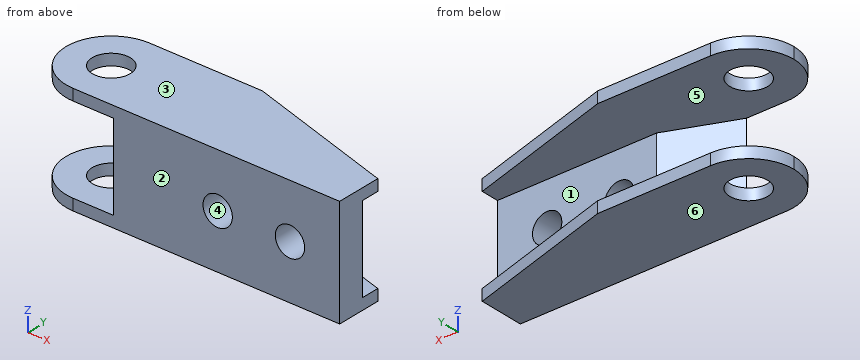
```python
from build123d import *

# Parameters (mm, degrees)
CROQUIS1_W              = 34.5
CROQUIS1_H              = 12
SALIENTE_EXTRUIR1_DEPTH = 10
REDONDEO1_R             = 5
CROQUIS8_W              = 34.5
CROQUIS8_H              = 9.5
CORTAR_EXTRUIR6_DEPTH   = 7
CROQUIS9_W              = 10.737065785
CROQUIS9_H              = 9.5
CORTAR_EXTRUIR7_DEPTH   = 21.822163672
CHAFL_N1_SIZE           = 3
CHAFL_N1_SIZE_2         = 7.42526056
CORTAR_EXTRUIR8_DEPTH   = 24.27149544
CROQUIS11_R             = 2.1
CORTAR_EXTRUIR9_DEPTH   = 24.27149544
CROQUIS12_R             = 1.625
CORTAR_EXTRUIR10_DEPTH  = 20.559204994


# Some blends are built 0.0001 mm under size
with BuildPart() as part:
    # Croquis1 → Saliente-Extruir1 (new body)
    with BuildSketch(Plane(origin=(0, 0, 0), x_dir=(1, 0, 0), z_dir=(0, 1, 0))):
        Rectangle(CROQUIS1_W, CROQUIS1_H)
    extrude(amount=SALIENTE_EXTRUIR1_DEPTH)

    # Redondeo1
    redondeo1_edges = [part.edges().sort_by_distance(p)[0] for p in [
        (-17.25, 10, 0),
        (-17.25, 0, 0),
    ]]
    fillet(redondeo1_edges, radius=REDONDEO1_R - 0.0001)  # a hair under: the kernel refuses the full size

    # Croquis8 → Cortar-Extruir6 (cut)
    with BuildSketch(Plane(origin=(0, 10, 0), x_dir=(1, 0, 0), z_dir=(0, 1, 0))):
        Rectangle(CROQUIS8_W, CROQUIS8_H)
    extrude(amount=-CORTAR_EXTRUIR6_DEPTH, mode=Mode.SUBTRACT)

    # Croquis9 → Cortar-Extruir7 (cut, through all)
    with BuildSketch(Plane.XZ):
        with Locations((-13.168532893, 0)):
            Rectangle(CROQUIS9_W, CROQUIS9_H)
    extrude(amount=-CORTAR_EXTRUIR7_DEPTH, mode=Mode.SUBTRACT)

    # Chaflán1
    # the kernel refuses this chamfer: 7.42526056, 3 mm, written as the material it takes off along each edge
    with BuildSketch(Plane(origin=(-7.8, 3, -4.75), x_dir=(-0.08816706473193606, -0.9961057015681392, 0), z_dir=(0, 0, 1))) as chafl_n1_piece_1:
        Polygon((CHAFL_N1_SIZE * 0.996105701568, CHAFL_N1_SIZE * 0.0881670647319), (-CHAFL_N1_SIZE_2 * 0.0881670647349, CHAFL_N1_SIZE_2 * 0.996105701602), (0, 0), align=None)
    extrude(amount=9.5, mode=Mode.SUBTRACT)

    # Croquis10 → Cortar-Extruir8 (cut, through all)
    with BuildSketch(Plane.XY.offset(6)):
        Polygon((0.25, 10), (17.25, 5), (17.25, 10), align=None)
    extrude(amount=-CORTAR_EXTRUIR8_DEPTH, mode=Mode.SUBTRACT)

    # Croquis11 → Cortar-Extruir9 (cut, through all)
    with BuildSketch(Plane.XY.offset(6)):
        with Locations((-12.25, 5)):
            Circle(CROQUIS11_R)
    extrude(amount=-CORTAR_EXTRUIR9_DEPTH, mode=Mode.SUBTRACT)

    # Croquis12 → Cortar-Extruir10 (cut, through all)
    with BuildSketch(Plane(origin=(0, 3, 0), x_dir=(1, 0, 0), z_dir=(0, 1, 0))):
        with Locations(Location((3.75, 0, 0), (0, 0, 270))):
            Circle(CROQUIS12_R)
        with Locations(Location((11.75, 0, 0), (0, 0, 270))):
            Circle(CROQUIS12_R)
    extrude(amount=-CORTAR_EXTRUIR10_DEPTH, mode=Mode.SUBTRACT)


solid = part.part
```
Geometry check sheet. Reference: the model listing, model coordinates, mm. Face numbers are marked on the shaded views. A direction names the side the tool comes from. Give positions to 0.01 mm unless a question says otherwise; leave off trailing zeros. Write each loop counter-clockwise with the first axis right and the second up, starting at its lowest first coordinate (ties: lowest second). Pieces come first, ordered by that corner, then holes. Notation, with made-up numbers: (-32.5, 11) - (23.5, 11) arc R23 ccw to (23.5, 43) - close; hole circle Ø7 at (32.5, 35). An arc over 180 degrees is marked (long way). Use a Markdown table: item, result.
Q1. Draft check along Z on the marked faces 1, 2, 3 and 4. Enter one of: pulls with the +Z half, pulls with the -Z half, needs draft (parallel to the pull), parting line crosses it, or undercut.
Computed:
| item | result |
|---|---|
| face 1 | undercut |
| face 2 | needs draft |
| face 3 | pulls with the +Z half |
| face 4 | undercut |
Q2. Section check A-A, the plane z = 0. Enter the section's corners in (x, y) (3 decimals), then the cut area to 3 significant figures.
Computed:
| item | result |
|---|---|
| outline | (-7.8, 0) - (2.125, 0) - (2.125, 3) - (-0.375, 3) - close; (5.375, 0) - (10.125, 0) - (10.125, 3) - (5.375, 3) - close; (13.375, 0) - (17.25, 0) - (17.25, 3) - (13.375, 3) - close |
| area | 44.5 mm² |
Q3. Go/stop test with flat-tipped pins: P1, Ø6, axis at x = 6.5, z = 2, coming from the -Y side; P2, Ø3, axis at y = 8, z = -4.5, coming from the -X side; P3, Ø3, axis at x = 6, z = 2, coming from the +Y side. Record where each tip stops, or that it passes through.
Computed:
| item | result |
|---|---|
| P1 | stops at y = 0 |
| P2 | stops at x = -17.01 |
| P3 | stops at y = 3 |
Q4. Section check C-C, the plane y = 8.5. Enter the section's corners in (x, z).
Computed:
| item | result |
|---|---|
| outline | (-15.82, -6) - (5.35, -6) - (5.35, -4.75) - (-15.82, -4.75) - close; (-15.82, 4.75) - (5.35, 4.75) - (5.35, 6) - (-15.82, 6) - close |
Q5. Section check D-D, the plane y = 4.25. Enter the section's corners in (x, z).
Computed:
| item | result |
|---|---|
| outline | (-17.19, -6) - (-14.21, -6) - (-14.21, -4.75) - (-17.19, -4.75) - close; (-17.19, 4.75) - (-14.21, 4.75) - (-14.21, 6) - (-17.19, 6) - close; (-10.29, -6) - (17.25, -6) - (17.25, -4.75) - (-10.29, -4.75) - close; (-10.29, 4.75) - (17.25, 4.75) - (17.25, 6) - (-10.29, 6) - close |
Q6. Section check B-B, the plane x = -8.5. Enter the section's corners in (y, z), then the cut area to 3 significant figures.
Computed:
| item | result |
|---|---|
| outline | (0, -6) - (10, -6) - (10, -4.75) - (0, -4.75) - close; (0, 4.75) - (10, 4.75) - (10, 6) - (0, 6) - close |
| area | 25.0 mm² |
Q7. Thickness scan on L1, parallel to Y at x = -12.25, z = -5; L2, parallel to X at y = 0.95, z = 0 (3 decimals); L3, parallel to Z at x = -15, y = 5.5. Record the ranges inside material, lowest first. Write a range as [from, to].
Computed:
| item | result |
|---|---|
| L1 | y = [0, 2.9], [7.1, 10] |
| L2 | x = [-5.449, 2.125], [5.375, 10.125], [13.375, 17.25] |
| L3 | z = [-6, -4.75], [4.75, 6] |
Q8. Set-up check for the marked faces 5 and 6: record each of +Z, -Z, +X, -X, +Y, -Y from which the full face is reachable in a straight line by a thin tool's end or side.
Computed:
| item | result |
|---|---|
| face 5 | -X, +Y |
| face 6 | -Z, +X, -X, +Y, -Y |
